Read the model definition and answer for the solid it produces. Units are mm, in the model's axes. A direction names the side the tool comes from. Coordinates: 2 decimals unless noted, no trailing zeros.
(1) Find the intervals of material crossed by probe 1 along X at (y, z) = (8.25, -107); probe 2 along Y at (x, z) = (135, 8.5); probe 3 along Z at (x, y) = (12.5, 7.5), in increasing order.
(2) The mould has two halves that part along Z. Classify faces 4 (the flat face through (9, 8, -115.608)), 5 (the flat face through (-24.13, 8, -27)), 6 (the flat face through (8, 5.08, -28)): +Z half, -Z half, draft (parallel to the pull), parting line (faces both ways), or undercut.
(3) Which of the six approach directions +Z, -Z, +X, -X, +Y, -Y give full straight-line access (tool end or side, diameter ignored) to faces 1 (the flat face through (9, 8, 60.101)), 2 (the flat face through (9, 8, 55.02)), 3 (the flat face through (43.18, 8, -27))?
(4) Given pin 1 (3 mm diameter, centred on y = 2.5, z = -105, fed in from -X); pin 2 (1.5 mm diameter, centred on y = 7, z = -7, fed in from -X); pin 3 (4 mm diameter, centred on x = 25, y = 8, fed in from -Z); pin 4 (12 mm diameter, centred on x = 36, z = -8, fed in from +Y), each flat-ended and moving along its own axis, determine where each tip first touches the part or whether it passes through.
from build123d import *

# Parameters (mm, degrees)
SKETCH1_W           = 201.6125
SKETCH1_H           = 201.6125
BOSS_EXTRUDE1_DEPTH = 5.08
BOSS_EXTRUDE1_TAPER = 33
SKETCH2_W           = 67.31
SKETCH2_H           = 175.708748127
SKETCH2_W_2         = 55.5625
SKETCH2_H_2         = 165.1
BOSS_EXTRUDE3_DEPTH = 5.08


with BuildPart() as part:
    # Sketch1 → Boss-Extrude1 (new body)
    with BuildSketch(Plane(origin=(0, 0, 0), x_dir=(1, 0, 0), z_dir=(0, 1, 0))):
        with Locations((55.240442456, 31.631215749)):
            Rectangle(SKETCH1_W, SKETCH1_H)
    extrude(amount=BOSS_EXTRUDE1_DEPTH, taper=BOSS_EXTRUDE1_TAPER)

    # Sketch2 → Boss-Extrude3 (add)
    with BuildSketch(Plane(origin=(0, 5.08, 0), x_dir=(1, 0, 0), z_dir=(0, 1, 0))):
        with Locations((9.525, 27.753321004)):
            Rectangle(SKETCH2_W, SKETCH2_H)
        with Locations((9.475412799, 27.530326262)):
            Rectangle(SKETCH2_W_2, SKETCH2_H_2, mode=Mode.SUBTRACT)
    extrude(amount=BOSS_EXTRUDE3_DEPTH)


solid = part.part
Response:
1. probe 1: x = -24.13 to -18.31, 37.26 to 43.18
1. probe 2: y = 0 to 5.08
1. probe 3: z = -115.61 to -110.08, 55.02 to 60.1
2. face 4: -Z half
2. face 5: draft
2. face 6: undercut
3. face 1: +Z, +X, -X, +Y
3. face 2: +Y
3. face 3: +Z, -Z, +X, +Y
4. pin 1: stops at x = -44.92
4. pin 2: stops at x = -24.13
4. pin 3: stops at z = -115.61
4. pin 4: stops at y = 10.16
